```python
from build123d import *

# Parameters (mm, degrees)
SKETCH1_W                                            = 335.8
SKETCH1_H                                            = 200
BOSS_EXTRUDE1_DEPTH                                  = 20
SKETCH2_W                                            = 275.8
SKETCH2_H                                            = 90
CUT_EXTRUDE1_DEPTH                                   = 197.44441962
SKETCH3_W                                            = 45
SKETCH3_H                                            = 90
CUT_EXTRUDE2_DEPTH                                   = 197.44441962
CBORE_FOR_M6_HEXAGON_SOCKET_HEAD_CAP_SCR_D           = 6.6
CBORE_FOR_M6_HEXAGON_SOCKET_HEAD_CAP_SCR_CBORE_D     = 11
CBORE_FOR_M6_HEXAGON_SOCKET_HEAD_CAP_SCR_CBORE_DEPTH = 6.8
M6_CLEARANCE_HOLE1_D                                 = 6.6
SKETCH8_W                                            = 20
SKETCH8_H                                            = 90
BOSS_EXTRUDE2_DEPTH                                  = 20
FILLET1_R                                            = 5
CBORE_FOR_M6_HEXAGON_SOCKET_HEAD_CAP_2_D             = 6.6
CBORE_FOR_M6_HEXAGON_SOCKET_HEAD_CAP_2_CBORE_D       = 11
CBORE_FOR_M6_HEXAGON_SOCKET_HEAD_CAP_2_CBORE_DEPTH   = 6.8
CHAMFER1_SIZE                                        = 10


with BuildPart() as part:
    # Sketch1 → Boss-Extrude1 (new body)
    with BuildSketch(Plane.XY):
        Rectangle(SKETCH1_W, SKETCH1_H)
    extrude(amount=BOSS_EXTRUDE1_DEPTH)

    # Sketch2 → Cut-Extrude1 (cut, through all)
    with BuildSketch(Plane.XY.offset(20)):
        with Locations((0, 25)):
            Rectangle(SKETCH2_W, SKETCH2_H)
    extrude(amount=-CUT_EXTRUDE1_DEPTH, mode=Mode.SUBTRACT)

    # Sketch3 → Cut-Extrude2 (cut, through all)
    with BuildSketch(Plane(origin=(0, 0, 0), x_dir=(-1, 0, 0), z_dir=(0, 0, -1))):
        with Locations((0, -10)):
            Rectangle(SKETCH3_W, SKETCH3_H)
    extrude(amount=-CUT_EXTRUDE2_DEPTH, mode=Mode.SUBTRACT)

    # CBORE for M6 Hexagon socket head cap scr (through all)
    with Locations(Plane.XY.offset(20)):
        with Locations((-142.9, -60), (-142.9, -90), (-82.9, -60), (-82.9, -90), (82.9, -90), (82.9, -60), (142.9, -90), (142.9, -60)):
            CounterBoreHole(CBORE_FOR_M6_HEXAGON_SOCKET_HEAD_CAP_SCR_D / 2, CBORE_FOR_M6_HEXAGON_SOCKET_HEAD_CAP_SCR_CBORE_D / 2, CBORE_FOR_M6_HEXAGON_SOCKET_HEAD_CAP_SCR_CBORE_DEPTH)

    # M6 Clearance Hole1 (through all)
    with Locations(Plane.XY.offset(20)):
        with Locations((0, -60), (0, -90)):
            Hole(M6_CLEARANCE_HOLE1_D / 2)

    # Sketch8 → Boss-Extrude2 (add)
    with BuildSketch(Plane.XY.offset(20)):
        with Locations((-32.5, 25)):
            Rectangle(SKETCH8_W, SKETCH8_H)
        with Locations((32.5, 25)):
            Rectangle(SKETCH8_W, SKETCH8_H)
    extrude(amount=-BOSS_EXTRUDE2_DEPTH)

    # Fillet1
    fillet1_edges = [part.edges().sort_by_distance(p)[0] for p in [
        (-22.5, 70, 10),
        (-42.5, -20, 10),
        (-42.5, 70, 10),
        (22.5, 70, 10),
        (42.5, 70, 10),
        (42.5, -20, 10),
        (-137.9, -20, 10),
        (-137.9, 70, 10),
        (137.9, 70, 10),
        (137.9, -20, 10),
        (22.5, -55, 10),
        (-22.5, -55, 10),
    ]]
    fillet(fillet1_edges, radius=FILLET1_R)

    # CBORE for M6 Hexagon socket head cap 2 (through all)
    with Locations(Plane.XY.offset(20)):
        with Locations((-152.9, 85), (-32.5, 60), (-32.5, 85), (32.5, 85), (32.5, 60), (152.9, 85)):
            CounterBoreHole(CBORE_FOR_M6_HEXAGON_SOCKET_HEAD_CAP_2_D / 2, CBORE_FOR_M6_HEXAGON_SOCKET_HEAD_CAP_2_CBORE_D / 2, CBORE_FOR_M6_HEXAGON_SOCKET_HEAD_CAP_2_CBORE_DEPTH)

    # Chamfer1
    chamfer1_edges = [part.edges().sort_by_distance(p)[0] for p in [
        (167.9, 100, 10),
        (-167.9, 100, 10),
    ]]
    chamfer(chamfer1_edges, length=CHAMFER1_SIZE)


solid = part.part
```
Part model, mm, in its own coordinate system. A direction names the side the tool comes from. Coordinates: 2 decimals unless noted, no trailing zeros. Write each loop counter-clockwise with the first axis right and the second up, starting at its lowest first coordinate (ties: lowest second). Pieces come first, ordered by that corner, then holes.
Item 1: Probe line 1 (X direction, y = 65, z = 1); line 2 (Y direction, x = 0, z = 10.75); line 3 (Y direction, x = 11, z = 13.5). List the from-to ranges inside material, lowest first.
Item 2: Slice it at A-A (x = -152.9). Write the cut outline in (y, z), and give its area (3 significant figures).
Item 3: Slice it at B-B (y = 46.5). Write the cut outline in (x, z), and give its area (3 significant figures).
Item 4: Slice it at D-D (x = -32.5). Write the cut outline in (y, z).
Item 5: Which spindle directions (+Z, -Z, +X, -X, +Y, -Y) get a long thin tool onto all of the face, cutting with end or side? Do faces 1 (the face through (-79.943, -85.362, 16.648)), 2 (the face through (0, -55, 10)). Say none if no direction does.
Item 6: Mould opens along Y. For faces 3 (the face through (30.726, 87.783, 6.508)), 4 (the face through (-2, -100, 10)) say: released by +Y, released by -Y, zero draft, split by the parting line, or undercut.
Item 7: Pin check, flat tips, straight feed: pin 1 (9 mm diameter, centred on x = -33.5, y = 84, fed in from +Z); pin 2 (3.5 mm diameter, centred on x = 34.5, y = 85.5, fed in from +Z). Stop position of each tip, or through.
Item 8: Slice it at C-C (x = -82.9). Write the cut outline in (y, z).
Results found:
1. line 1: x = -167.9 to -137.9, -42.5 to -22.5, 22.5 to 42.5, 137.9 to 167.9
1. line 2: y = -100 to -93.3, -86.7 to -63.3, -56.7 to -55, 70 to 100
1. line 3: y = -100 to -55, 70 to 100
2. outline: (-100, 0) - (81.7, 0) - (81.7, 13.2) - (79.5, 13.2) - (79.5, 20) - (-100, 20) - close; (88.3, 0) - (100, 0) - (100, 20) - (90.5, 20) - (90.5, 13.2) - (88.3, 13.2) - close
2. area: 3,840 mm2
3. outline: (-167.9, 0) - (-137.9, 0) - (-137.9, 20) - (-167.9, 20) - close; (-42.5, 0) - (-22.5, 0) - (-22.5, 20) - (-42.5, 20) - close; (22.5, 0) - (42.5, 0) - (42.5, 20) - (22.5, 20) - close; (137.9, 0) - (167.9, 0) - (167.9, 20) - (137.9, 20) - close
3. area: 2,000 mm2
4. outline: (-100, 0) - (56.7, 0) - (56.7, 13.2) - (54.5, 13.2) - (54.5, 20) - (-100, 20) - close; (63.3, 0) - (81.7, 0) - (81.7, 13.2) - (79.5, 13.2) - (79.5, 20) - (65.5, 20) - (65.5, 13.2) - (63.3, 13.2) - close; (88.3, 0) - (100, 0) - (100, 20) - (90.5, 20) - (90.5, 13.2) - (88.3, 13.2) - close
5. face 1: +Z
5. face 2: +Z, -Z
6. face 3: undercut
6. face 4: released by -Y
7. pin 1: stops at z = 20
7. pin 2: stops at z = 13.2
8. outline: (-100, 0) - (-93.3, 0) - (-93.3, 13.2) - (-95.5, 13.2) - (-95.5, 20) - (-100, 20) - close; (-86.7, 0) - (-63.3, 0) - (-63.3, 13.2) - (-65.5, 13.2) - (-65.5, 20) - (-84.5, 20) - (-84.5, 13.2) - (-86.7, 13.2) - close; (-56.7, 0) - (-20, 0) - (-20, 20) - (-54.5, 20) - (-54.5, 13.2) - (-56.7, 13.2) - close; (70, 0) - (100, 0) - (100, 20) - (70, 20) - close
